```python
from build123d import *

# Parameters (mm, degrees)
SKETCH_W        = 54
SKETCH_H        = 54
PAD_DEPTH       = 2
SKETCH001_R     = 1.27
SKETCH001_R_2   = 6.25
SKETCH001_W     = 32
SKETCH001_H     = 16
POCKET_DEPTH    = 2
CHAMFER_SIZE    = 1
SKETCH006_W     = 4
SKETCH006_H     = 13
SKETCH006_H_2   = 3
POCKET004_DEPTH = 1


with BuildPart() as part:
    # Sketch → Pad (new body)
    with BuildSketch(Plane.XY):
        Rectangle(SKETCH_W, SKETCH_H)
    extrude(amount=PAD_DEPTH)

    # Sketch001 (on Face6 of Pad) → Pocket (cut)
    with BuildSketch(Plane.XY.offset(2)):
        with Locations((-22.86, -4)):
            Circle(SKETCH001_R)
        with Locations((22.86, -4)):
            Circle(SKETCH001_R)
        with Locations((22.86, -21.78)):
            Circle(SKETCH001_R)
        with Locations((-22.86, -21.78)):
            Circle(SKETCH001_R)
        with Locations((-12.5, 18)):
            Circle(SKETCH001_R_2)
        with Locations((12.5, 18)):
            Circle(SKETCH001_R_2)
        with Locations((0.64, -12.89)):
            Rectangle(SKETCH001_W, SKETCH001_H)
    extrude(amount=-POCKET_DEPTH, mode=Mode.SUBTRACT)

    # Chamfer
    chamfer_edges = [part.edges().sort_by_distance(p)[0] for p in [
        (0.64, -20.89, 2),
        (-15.36, -12.89, 2),
        (0.64, -4.89, 2),
        (16.64, -12.89, 2),
    ]]
    chamfer(chamfer_edges, length=CHAMFER_SIZE)

    # Sketch006 (on Face20 of Chamfer) → Pocket004 (cut)
    with BuildSketch(Plane(origin=(0, 0, 0), x_dir=(1, 0, 0), z_dir=(0, 0, -1))):
        with Locations((-20.8, 13)):
            Rectangle(SKETCH006_W, SKETCH006_H)
        with Locations((-18.5, 3.7)):
            Rectangle(SKETCH006_W, SKETCH006_H_2)
    extrude(amount=-POCKET004_DEPTH, mode=Mode.SUBTRACT)


solid = part.part
```
CAD build for the part. Positions are in the model's coordinates, mm. A direction names the side the tool comes from. Round coordinates to 2 decimals unless told otherwise and drop trailing zeros. Loops run counter-clockwise (first coordinate to the right, second up) from the corner with the lowest first, then second, coordinate; pieces in that order, holes last. Notation, with made-up numbers: (57.25, 50.25) - (109.25, 50.25) arc R29 ccw to (109.25, 74.25) - close; hole circle Ø3 at (-19, 19.5). An arc over 180 degrees is marked (long way). Return JSON: item names as keys, results as strings. Group by question number.
Q1. Band-saw the part on A-A on x = 0.5. Give the cut face in (y, z), plus the area to 3 significant figures.
Q2. Tool access for faces 1 (the face through (22.58, -5.24, 1.01)), 2 (the face through (-19, -4, 1)): list every direction of +Z, -Z, +X, -X, +Y, -Y with a clear straight run to the whole face (end or side of a thin tool).
Q3. Band-saw the part on D-D on z = 1.6. Give the cut face in (x, y).
Q4. Drill centre lines: line 1 along Y through (x, z) = (-19.5, 0.35); line 2 along Y through (x, z) = (22.86, 0.5); line 3 along X through (y, z) = (19, 1.45). Where is each one in solid material? Low to high. Write a range as [from, to].
Q5. Two-plate mould, pull along X, no slides. Class faces 3 (the face through (22.58, -23.02, 1.01)), 4 (the face through (0, 0, 2)), 5 (the face through (-27, 0, 1)), 6 (the face through (-17.46, 14.2, 1.01)): +X half, -X half, draft (parallel to the pull), parting line (faces both ways), or undercut.
Q6. Band-saw the part on B-B on x = 12.5. Give the cut face in (y, z), plus the area to 3 significant figures.
Q7. Flat gauge pins, fed straight in: pin 1 Ø7.5 at (x, y) = (-12.5, 18) entering from -Z; pin 2 Ø1.2 at (x, y) = (-20.5, -10) entering from -Z. Where does each tip first touch, or does it go through?
Q8. Band-saw the part on C-C on y = 18. Give the cut face in (x, z), plus the area to 3 significant figures.
Solutions:
{
 "1": {"outline": "(-27, 0) - (-20.89, 0) - (-20.89, 1) - (-21.89, 2) - (-27, 2) - close; (-4.89, 0) - (27, 0) - (27, 2) - (-3.89, 2) - (-4.89, 1) - close", "area": "75.0 mm^2"},
 "2": {"face 1": "+Z, -Z", "face 2": "-Z"},
 "3": {"outline": "(-27, -27) - (27, -27) - (27, 27) - (-27, 27) - close; hole circle Ø2.54 at (-22.86, -21.78); hole circle Ø2.54 at (-22.86, -4); hole circle Ø12.5 at (-12.5, 18); hole (-15.96, -21.49) - (17.24, -21.49) - (17.24, -4.29) - (-15.96, -4.29) - close; hole circle Ø12.5 at (12.5, 18); hole circle Ø2.54 at (22.86, -21.78); hole circle Ø2.54 at (22.86, -4)"},
 "4": {"line 1": "y = [-27, -19.5], [-6.5, -5.2], [-2.2, 27]", "line 2": "y = [-27, -23.05], [-20.51, -5.27], [-2.73, 27]", "line 3": "x = [-27, -18.67], [-6.33, 6.33], [18.67, 27]"},
 "5": {"face 3": "undercut", "face 4": "draft", "face 5": "-X half", "face 6": "undercut"},
 "6": {"outline": "(-27, 0) - (-20.89, 0) - (-20.89, 1) - (-21.89, 2) - (-27, 2) - close; (-4.89, 0) - (11.75, 0) - (11.75, 2) - (-3.89, 2) - (-4.89, 1) - close; (24.25, 0) - (27, 0) - (27, 2) - (24.25, 2) - close", "area": "50.0 mm^2"},
 "7": {"pin 1": "passes through", "pin 2": "stops at z = 1"},
 "8": {"outline": "(-27, 0) - (-18.75, 0) - (-18.75, 2) - (-27, 2) - close; (-6.25, 0) - (6.25, 0) - (6.25, 2) - (-6.25, 2) - close; (18.75, 0) - (27, 0) - (27, 2) - (18.75, 2) - close", "area": "58.0 mm^2"}
}
